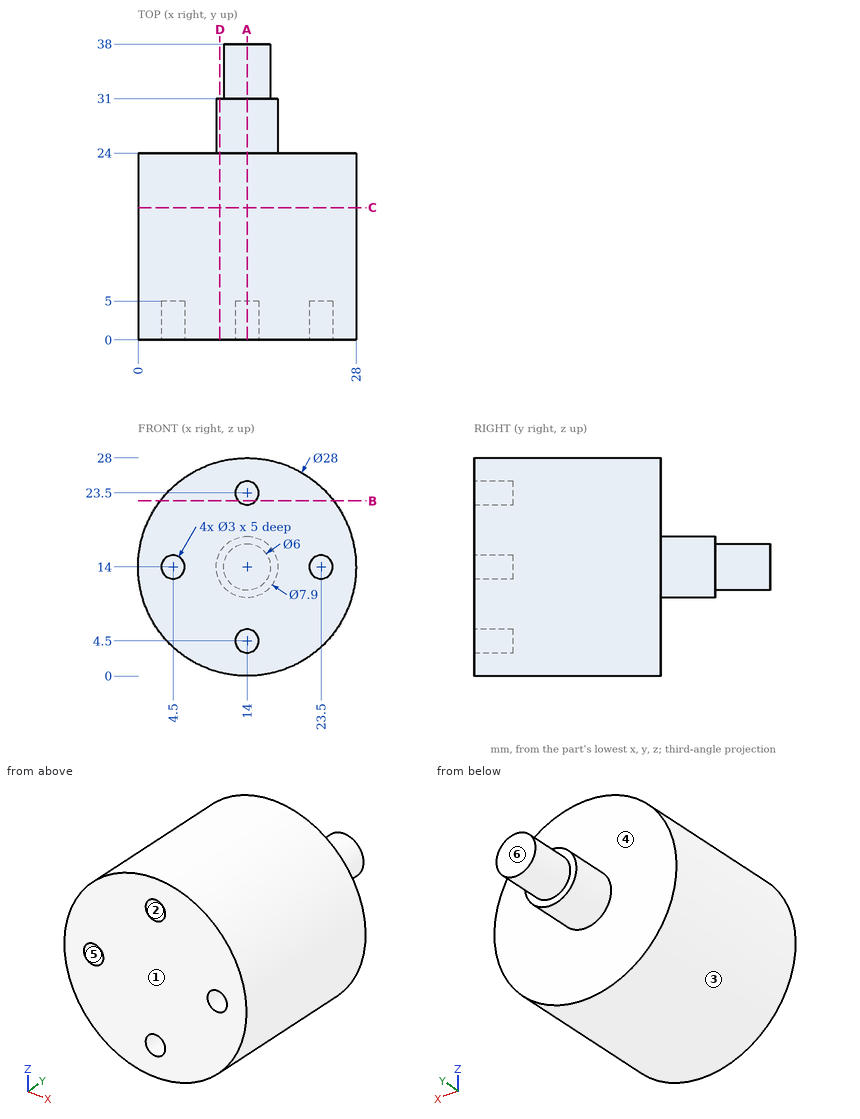
Here's the drawing with two shaded views (mm, measured from the low corner). I have some questions. A direction names the side the tool comes from. Coordinates: 2 decimals unless noted, no trailing zeros. Order: outer loops, then holes, each group sorted by start corner. A loop starts at its lowest first (then second) coordinate and runs counter-clockwise, first axis right, second up.
Item 1: For the marked faces 4, 5 and 6, which set-ups out of +Z, -Z, +X, -X, +Y, -Y let a thin tool reach every point of the face, with its end or its side?
Result sheet:
face 4: +Y
face 5: -Y
face 6: +Z, -Z, +X, -X, +Y
Item 2: If we section it at B-B on z = 22.5: List the corners of the cut face in (x, y) for me, plus the area to 3 significant figures.
Result sheet:
outline: (2.88, 0) - (12.88, 0) - (12.88, 5) - (15.12, 5) - (15.12, 0) - (25.12, 0) - (25.12, 24) - (2.88, 24) - close
area: 523 mm2
Item 3: If we section it at D-D on x = 10.5: List the corners of the cut face in (y, z) for me, plus the area to 3 significant figures.
Result sheet:
outline: (0, 0.44) - (24, 0.44) - (24, 12.17) - (31, 12.17) - (31, 15.83) - (24, 15.83) - (24, 27.56) - (0, 27.56) - close
area: 676 mm2
Item 4: If we mould it in two halves opening along Z, with no side actions, what happens to the marked faces 1, 2 and 3? For each: +Z half, -Z half, draft (parallel to the pull), parting line (faces both ways), or undercut.
Result sheet:
face 1: draft
face 2: undercut
face 3: parting line
Item 5: For P1, Ø1.8, axis at x = 14, z = 23.5, coming from the +Y side; P2, Ø8, axis at x = 14.5, z = 10, coming from the -Y side; P3, Ø1.8, axis at x = 4.5, z = 14, coming from the -Y side; P4, Ø8, axis at x = 7, y = 17.5, coming from the -Z side, each with a flat end and sliding along its axis, tell me the tip position at first contact or that it passes through.
Result sheet:
P1: stops at y = 24
P2: stops at y = 0
P3: stops at y = 5
P4: stops at z = 0.33
Item 6: I need wall thicknesses on line 1 (X direction, y = 3.65, z = 14); line 2 (Y direction, x = 7.75, z = 21.75); line 3 (Y direction, x = 11, z = 13.5). Which ranges of each line are inside material? Lowest first, please.
Result sheet:
line 1: x = 0 to 3, 6 to 22, 25 to 28
line 2: y = 0 to 24
line 3: y = 0 to 31
Item 7: If we section it at A-A on x = 14: List the corners of the cut face in (y, z) for me.
Result sheet:
outline: (0, 0) - (24, 0) - (24, 10.05) - (31, 10.05) - (31, 11) - (38, 11) - (38, 17) - (31, 17) - (31, 17.95) - (24, 17.95) - (24, 28) - (0, 28) - (0, 25) - (5, 25) - (5, 22) - (0, 22) - (0, 6) - (5, 6) - (5, 3) - (0, 3) - close
Item 8: If we section it at C-C on y = 17: List the corners of the cut face in (x, z) for me, plus the area to 3 significant figures.
Result sheet:
outline: circle Ø28 at (14, 14)
area: 616 mm2
